```python
from build123d import *

# Parameters (mm, degrees)
F0_R     = 3.500564
F1_DEPTH = 6.35


with BuildPart() as f1:
    # F0 (on Top) → F1 (new body)
    with BuildSketch(Plane.XY):
        with BuildLine():
            Line((-9.096524, 12.534158), (-28.146524, 12.534158))
            ThreePointArc((-28.146524, 12.534158), (-34.413602, 6.267079), (-28.146524, 0))
            Line((-28.146524, 0), (-9.096524, 0))
            ThreePointArc((-9.096524, 0), (-2.829445, 6.267079), (-9.096524, 12.534158))
        make_face()
        with Locations((-18.621524, 6.01799)):
            Circle(F0_R, mode=Mode.SUBTRACT)
    extrude(amount=F1_DEPTH)


solid = f1.part
```
Source: CAD feature listing. Evaluate the final solid. Frame: model axes, mm. Give positions to 0.01 mm unless a question says otherwise; leave off trailing zeros. Loops run counter-clockwise (first coordinate to the right, second up) from the corner with the lowest first, then second, coordinate; pieces in that order, holes last. Notation, with made-up numbers: (24.25, 0) - (38.25, 0) arc R27 ccw to (38.25, 26) - close; hole circle Ø11 at (-16, -39.5). An arc over 180 degrees is marked (long way). Use CSV: the item, a comma, the result in double quotes. Start each with the question number.
1. Ray query, L1, parallel to X at y = 6, z = 4; L2, parallel to Y at x = -15.5, z = 2.25; L3, parallel to Y at x = -19, z = 3. Return the intervals inside material, ascending.
2. Section A-A (x = -21.5). Output: boundary loops of the cut face in (y, z).
3. Draft query along X for faces 1 (the cylindrical face through (-34.412, 6.405, 3.131)), 2 (the cylindrical face through (-2.83, 6.13, 3.13)), 3 (the cylindrical face through (-22.12, 6.17, 3.13)), 4 (the flat face through (-22.4, 6.4, 6.35)). Return one class per face: +X half, -X half, draft (parallel to the pull), parting line (faces both ways), or undercut.
4. Section D-D (x = -32). Output: boundary loops of the cut face in (y, z), then the cut area to 3 significant figures.
5. Section C-C (y = 11.75). Output: boundary loops of the cut face in (x, z).
Response:
1,L1,"-34.41 to -22.12, -15.12 to -2.84"
1,L2,"0 to 4.43, 7.6 to 12.53"
1,L3,"0 to 2.54, 9.5 to 12.53"
2,outline,"(0, 0) - (4.03, 0) - (4.03, 6.35) - (0, 6.35) - close; (8.01, 0) - (12.53, 0) - (12.53, 6.35) - (8.01, 6.35) - close"
3,face 1,"-X half"
3,face 2,"+X half"
3,face 3,"undercut"
3,face 4,"draft"
4,outline,"(1.32, 0) - (11.21, 0) - (11.21, 6.35) - (1.32, 6.35) - close"
4,area,"62.8 mm²"
5,outline,"(-31.18, 0) - (-6.06, 0) - (-6.06, 6.35) - (-31.18, 6.35) - close"
